Geometry: final body of the model. Coordinates: model frame, mm. A direction names the side the tool comes from. Coordinates: 2 decimals unless noted, no trailing zeros. Order: outer loops, then holes, each group sorted by start corner. A loop starts at its lowest first (then second) coordinate and runs counter-clockwise, first axis right, second up. Notation, with made-up numbers: (45.25, 23.25) - (86.25, 23.25) arc R19 cw to (86.25, 42.25) - close; hole circle Ø5 at (50.25, -26). An arc over 180 degrees is marked (long way). Use a Markdown table: item, result. Add a question column.
```python
from build123d import *

# Parameters (mm, degrees)
SKETCH1_R           = 15
BOSS_EXTRUDE1_DEPTH = 3
BOSS_EXTRUDE2_DEPTH = 3
CIRPATTERN1_COUNT   = 40
SKETCH4_R           = 3.2
CUT_EXTRUDE1_DEPTH  = 3
SKETCH5_R           = 1
CUT_EXTRUDE2_DEPTH  = 3


with BuildPart() as part:
    # Sketch1 → Boss-Extrude1 (new body)
    with BuildSketch(Plane(origin=(0, 0, 0), x_dir=(1, 0, 0), z_dir=(0, 1, 0))):
        with Locations(Location((0, 0, 0), (0, 0, 270))):
            Circle(SKETCH1_R)
    extrude(amount=BOSS_EXTRUDE1_DEPTH)

    # Sketch3 → Boss-Extrude2 (add)
    with BuildSketch(Plane(origin=(0, 3, 0), x_dir=(1, 0, 0), z_dir=(0, 1, 0))):
        Polygon((-1, 14.8), (-0.25, 17.8), (0.25, 17.8), (1, 14.8), align=None)
    boss_extrude2 = extrude(amount=-BOSS_EXTRUDE2_DEPTH)

    # CirPattern1: Boss-Extrude2 ×40 about axis
    cirpattern1_axis = Axis((0, 0, 0), (0, 1, 0))
    for i in range(1, CIRPATTERN1_COUNT):
        add(boss_extrude2.rotate(cirpattern1_axis, i * 360 / CIRPATTERN1_COUNT))

    # Sketch4 → Cut-Extrude1 (cut)
    with BuildSketch(Plane(origin=(0, 3, 0), x_dir=(1, 0, 0), z_dir=(0, 1, 0))):
        with Locations(Location((0, 0, 0), (0, 0, 270))):
            Circle(SKETCH4_R)
    extrude(amount=-CUT_EXTRUDE1_DEPTH, mode=Mode.SUBTRACT)

    # Sketch5 → Cut-Extrude2 (cut)
    with BuildSketch(Plane(origin=(0, 3, 0), x_dir=(1, 0, 0), z_dir=(0, 1, 0))):
        with Locations(Location((2, -7.5, 0), (0, 0, 270))):
            Circle(SKETCH5_R)
        with Locations(Location((5, -10.5, 0), (0, 0, 270))):
            Circle(SKETCH5_R)
    extrude(amount=-CUT_EXTRUDE2_DEPTH, mode=Mode.SUBTRACT)


solid = part.part
```
1) Section A-A (z = -2). Return loops of the section in (x, y).
2) Set-up query: faces 5 (the face through (-7.97, 1.52, -14.3)), 6 (the face through (-0.6, 1.5, -16.4)), 7 (the face through (16.109, 1.521, 3.158)). Return all of +Z, -Z, +X, -X, +Y, -Y with unobstructed straight access to the full face (end or side cutting, diameter ignored); none if empty.
3) Section D-D (z = -6.5). Return loops of the section in (x, y), then the cut area to 3 significant figures.
4) Section B-B (x = 2). Return loops of the section in (y, z).
5) Section C-C (y = 2.35). Give the number of separate pieces and of enclosed holes in the cut face, then the cut area to 3 significant figures.
6) Ray query, line 1 along Z through (x, y) = (-1, 2.75); line 2 along Z through (x, y) = (12, 1.9); line 3 along X through (y, z) = (1.35, 10.5). Return the intervals inside material, ascending.
7) Pin query (flat end, axial travel): pin 1 (1.5 mm diameter, centred on y = 2.5, z = 4, fed in from -X); pin 2 (1.5 mm diameter, centred on y = 1, z = -12, fed in from -X). Return the tip coordinate at first contact, or that it passes through.
8) Draft query along X for faces 1 (the face through (15.79, 1.52, -4.5)), 2 (the face through (15.376, 1.521, -5.636)), 3 (the face through (-15.79, 1.52, 4.5)), 4 (the face through (9.158, 1.521, 13.624)). Return one class per face: pulls with the +X half, pulls with the -X half, needs draft (parallel to the pull), parting line crosses it, or undercut.
Values follow:
| question | item | result |
|---|---|---|
| 1 | outline | (-16.36, 0) - (-2.5, 0) - (-2.5, 3) - (-16.36, 3) - close; (2.5, 0) - (16.36, 0) - (16.36, 3) - (2.5, 3) - close |
| 2 | face 5 | +Y, -Y |
| 2 | face 6 | -Z, +Y, -Y |
| 2 | face 7 | +X, +Y, -Y |
| 3 | outline | (-14.41, 0) - (14.41, 0) - (14.41, 3) - (-14.41, 3) - close |
| 3 | area | 86.5 mm² |
| 4 | outline | (0, -16.36) - (3, -16.36) - (3, -2.5) - (0, -2.5) - close; (0, 2.5) - (3, 2.5) - (3, 6.5) - (0, 6.5) - close; (0, 8.5) - (3, 8.5) - (3, 16.36) - (0, 16.36) - close |
| 5 | separate pieces | 1 |
| 5 | enclosed holes | 3 |
| 5 | area | 804 mm² |
| 6 | line 1 | z = -14.97 to -3.04, 3.04 to 14.97 |
| 6 | line 2 | z = -12.52 to -11.14, -9.76 to 9.76, 11.14 to 12.52 |
| 6 | line 3 | x = -14.37 to -13.84, -11.62 to 4, 6 to 11.62, 13.84 to 14.37 |
| 7 | pin 1 | stops at x = -16.19 |
| 7 | pin 2 | stops at x = -12.76 |
| 8 | face 1 | pulls with the +X half |
| 8 | face 2 | undercut |
| 8 | face 3 | pulls with the -X half |
| 8 | face 4 | undercut |
